Read the model definition and answer for the solid it produces. Units are mm, in the model's axes. Give positions to 0.01 mm unless a question says otherwise; leave off trailing zeros. Write each loop counter-clockwise with the first axis right and the second up, starting at its lowest first coordinate (ties: lowest second). Pieces come first, ordered by that corner, then holes. Notation, with made-up numbers: M 59.25,-1 L 111.25,-1 A18 cw 111.25,3 Z; hole C 71,26 d5. An arc over 180 degrees is marked long. Use a Markdown table: item, result. Add a question column.
Item 1: A cutting plane is placed at C-C on y = 42. Determine the outline of the cut face in (x, z), then the cut area to 3 significant figures.
Item 2: A cutting plane is placed at A-A on y = -99. Determine the outline of the cut face in (x, z).
Item 3: Consider probe 1 along Y at (x, z) = (3.15, 0); probe 2 along Z at (x, y) = (5.7, 95.5); probe 3 along Y at (x, z) = (4.3, 29.5). Determine where each line is inside the solid, lowest interval first. Write a range as [from, to].
Item 4: A cutting plane is placed at B-B on x = 1.4. Count the separate pieces of the cut face and the enclosed holes in it, then the cut area to 3 significant figures.
Item 5: Given P1, Ø1.8, axis at x = 2.5, z = 59.5, coming from the -Y side; P2, Ø1.8, axis at x = 1.5, y = -123.5, coming from the +Z side; P3, Ø3, axis at x = 2.5, z = -59.5, coming from the +Y side, each flat-ended and moving along its own axis, determine where each tip first touches the part or whether it passes through.
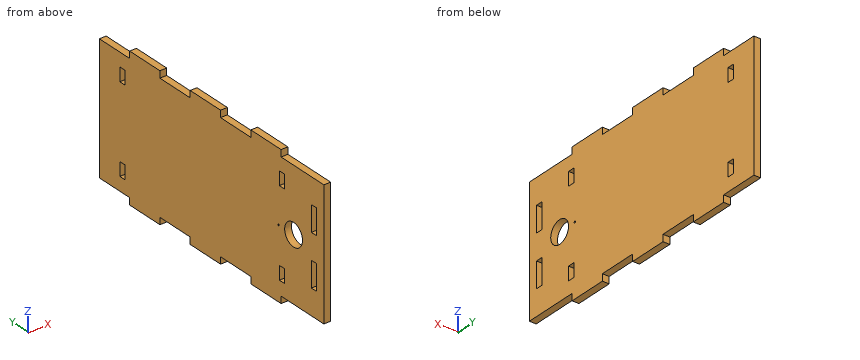
from build123d import *

# Parameters (mm, degrees)
SKETCH1_W           = 112.5
SKETCH1_H           = 238
BOSS_EXTRUDE1_DEPTH = 6
SKETCH2_R           = 10
SKETCH2_R_2         = 0.75
CUT_EXTRUDE1_DEPTH  = 6
SKETCH3_W           = 12
SKETCH3_H           = 6
CUT_EXTRUDE2_DEPTH  = 6
SKETCH4_W           = 6
SKETCH4_H           = 22.5
BOSS_EXTRUDE2_DEPTH = 6
SKETCH5_W           = 12
SKETCH5_H           = 6
CUT_EXTRUDE3_DEPTH  = 6
SKETCH6_W           = 6
SKETCH6_H           = 34
BOSS_EXTRUDE3_DEPTH = 6
SKETCH7_W           = 6
SKETCH7_H           = 112.5
BOSS_EXTRUDE4_DEPTH = 8


with BuildPart() as part:
    # Sketch1 → Boss-Extrude1 (new body)
    with BuildSketch(Plane(origin=(0, 0, 0), x_dir=(0, 0, -1), z_dir=(1, 0, 0))):
        Rectangle(SKETCH1_W, SKETCH1_H)
    extrude(amount=BOSS_EXTRUDE1_DEPTH)

    # Sketch2 → Cut-Extrude1 (cut)
    with BuildSketch(Plane(origin=(6, 0, 0), x_dir=(0, 0, -1), z_dir=(1, 0, 0))):
        with Locations((0, -99)):
            Circle(SKETCH2_R)
        with Locations((0, -82.029437252)):
            Circle(SKETCH2_R_2)
    extrude(amount=-CUT_EXTRUDE1_DEPTH, mode=Mode.SUBTRACT)

    # Sketch3 → Cut-Extrude2 (cut)
    with BuildSketch(Plane(origin=(6, 0, 0), x_dir=(0, 0, -1), z_dir=(1, 0, 0))):
        with Locations((-38.25, -86)):
            Rectangle(SKETCH3_W, SKETCH3_H)
        with Locations((38.25, -86)):
            Rectangle(SKETCH3_W, SKETCH3_H)
    extrude(amount=-CUT_EXTRUDE2_DEPTH, mode=Mode.SUBTRACT)

    # Sketch4 → Boss-Extrude2 (add)
    with BuildSketch(Plane.XZ.offset(119)):
        with Locations((3, -45)):
            Rectangle(SKETCH4_W, SKETCH4_H)
        with Locations((3, 0)):
            Rectangle(SKETCH4_W, SKETCH4_H)
        with Locations((3, 45)):
            Rectangle(SKETCH4_W, SKETCH4_H)
    extrude(amount=BOSS_EXTRUDE2_DEPTH)

    # Sketch5 → Cut-Extrude3 (cut)
    with BuildSketch(Plane(origin=(6, 0, 0), x_dir=(0, 0, -1), z_dir=(1, 0, 0))):
        with Locations((-38.25, 93)):
            Rectangle(SKETCH5_W, SKETCH5_H)
        with Locations((38.25, 93)):
            Rectangle(SKETCH5_W, SKETCH5_H)
    extrude(amount=-CUT_EXTRUDE3_DEPTH, mode=Mode.SUBTRACT)

    # Sketch6 → Boss-Extrude3 (add)
    with BuildSketch(Plane(origin=(0, 0, -56.25), x_dir=(-1, 0, 0), z_dir=(0, 0, -1))):
        with Locations((-3, 68)):
            Rectangle(SKETCH6_W, SKETCH6_H)
        with Locations((-3, 0)):
            Rectangle(SKETCH6_W, SKETCH6_H)
        with Locations((-3, -68)):
            Rectangle(SKETCH6_W, SKETCH6_H)
    boss_extrude3 = extrude(amount=BOSS_EXTRUDE3_DEPTH)

    # Mirror1: Boss-Extrude3 across plane
    add(boss_extrude3.mirror(Plane.XY))

    # Sketch7 → Boss-Extrude4 (add)
    with BuildSketch(Plane(origin=(0, -125, 0), x_dir=(-1, 0, 0), z_dir=(0, -1, 0))):
        with Locations((-3, 0)):
            Rectangle(SKETCH7_W, SKETCH7_H)
    extrude(amount=BOSS_EXTRUDE4_DEPTH)


solid = part.part
Filled in:
| question | item | result |
|---|---|---|
| 1 | outline | M 0,-56.25 L 6,-56.25 L 6,56.25 L 0,56.25 Z |
| 1 | area | 675 mm² |
| 2 | outline | M 0,-56.25 L 6,-56.25 L 6,-10 L 0,-10 Z; M 0,10 L 6,10 L 6,56.25 L 0,56.25 Z |
| 3 | probe 1 | [-133, -109], [-89, -82.78], [-81.28, 119] |
| 3 | probe 2 | [-56.25, -44.25], [-32.25, 32.25], [44.25, 56.25] |
| 3 | probe 3 | [-133, -125], [-119, 119] |
| 4 | separate pieces | 1 |
| 4 | enclosed holes | 8 |
| 4 | area | 28,700 mm² |
| 5 | P1 | y = -85 |
| 5 | P2 | z = 56.25 |
| 5 | P3 | y = 85 |
